```python
from build123d import *

# Parameters (mm, degrees)
SKETCH1_W                       = 45
SKETCH1_H                       = 20
SKETCH1_R                       = 4.9235
BOSS_EXTRUDE1_DEPTH             = 12.7
TAP_DRILL_FOR_M3X0_5_TAP1_D     = 2.584625
TAP_DRILL_FOR_M3X0_5_TAP1_DEPTH = 10
TAP_DRILL_FOR_M3X0_5_TAP1_TIP   = 0.776499689
FILLET1_R                       = 2
CHAMFER1_SIZE                   = 0.5


with BuildPart() as part:
    # Sketch1 → Boss-Extrude1 (new body)
    with BuildSketch(Plane.XY):
        with Locations((5.818965517, -6.284482759)):
            Rectangle(SKETCH1_W, SKETCH1_H)
        with Locations((-6.681034483, -8.784482759)):
            Circle(SKETCH1_R, mode=Mode.SUBTRACT)
        with Locations((18.318965517, -8.784482759)):
            Circle(SKETCH1_R, mode=Mode.SUBTRACT)
    extrude(amount=BOSS_EXTRUDE1_DEPTH)

    # Tap Drill for M3x0.5 Tap1
    with Locations(Plane.XY.offset(12.7)):
        with Locations((5.818965517, -6.284482759), (5.818965517, -11.284482759)):
            Hole(TAP_DRILL_FOR_M3X0_5_TAP1_D / 2, depth=TAP_DRILL_FOR_M3X0_5_TAP1_DEPTH)
            with Locations((0, 0, -(TAP_DRILL_FOR_M3X0_5_TAP1_DEPTH + TAP_DRILL_FOR_M3X0_5_TAP1_TIP / 2))):  # 118° drill point
                Cone(0, TAP_DRILL_FOR_M3X0_5_TAP1_D / 2, TAP_DRILL_FOR_M3X0_5_TAP1_TIP, mode=Mode.SUBTRACT)

    # Fillet1
    fillet1_edges = [part.edges().sort_by_distance(p)[0] for p in [
        (-16.681034483, 3.715517241, 6.35),
        (28.318965517, 3.715517241, 6.35),
        (28.318965517, -16.284482759, 6.35),
        (-16.681034483, -16.284482759, 6.35),
    ]]
    fillet(fillet1_edges, radius=FILLET1_R)

    # Sketch8 → Tap Drill for M3x0.5 Tap2 (revolve, cut)
    with BuildSketch(Plane(origin=(-16.681034483, -3.784482759, 2.5), x_dir=(0, 0, 1), z_dir=(0, 1, 0))):
        Polygon((0, 0), (0, 5.776499689), (1.2923125, 5), (1.2923125, 0), align=None)
    tap_drill_for_m3x0_5_tap2 = revolve(axis=Axis((-23.031034483, -3.784482759, 2.5), (1, 0, 0)), mode=Mode.SUBTRACT)

    # Mirror3: Tap Drill for M3x0.5 Tap2 across plane
    add(tap_drill_for_m3x0_5_tap2.mirror(Plane(origin=(5.818965517, 0, 0), x_dir=(0, 0, 1), z_dir=(1, 0, 0))), mode=Mode.SUBTRACT)

    # Chamfer1
    chamfer1_edges = [part.edges().sort_by_distance(p)[0] for p in [
        (-16.681034483, -3.784482759, 1.2076875),
        (28.318965517, -3.784482759, 1.2076875),
    ]]
    chamfer(chamfer1_edges, length=CHAMFER1_SIZE)


solid = part.part
```
CAD build for the part. Positions are in the model's coordinates, mm. A direction names the side the tool comes from. Coordinates: 2 decimals unless noted, no trailing zeros. Write each loop counter-clockwise with the first axis right and the second up, starting at its lowest first coordinate (ties: lowest second). Pieces come first, ordered by that corner, then holes.
(1) Two-plate mould, pull along Y, no slides. Class faces 5 (the face through (5.77, -11.504, 2.058)), 6 (the face through (-16.111, 3.114, 6.439)), 7 (the face through (6, -4, 12.7)): +Y half, -Y half, draft (parallel to the pull), parting line (faces both ways), or undercut.
(2) Cut at A-A, the plane z = 9.75. List the corners of the cut face in (x, y).
(3) Flat gauge pins, fed straight in: pin 1 (2.5 mm diameter, centred on y = -3.78, z = 2.5, fed in from +X); pin 2 (3.5 mm diameter, centred on y = -3.78, z = 2.5, fed in from -X). Where does each tip first touch, or does it go through?
(4) Cut at C-C, the plane x = -13. List the corners of the cut face in (y, z).
(5) Cut at D-D, the plane y = -7. Count the separate pieces of the cut face and the enclosed holes in it, and give its area (3 significant figures).
(6) Cut at B-B, the plane x = -5. List the corners of the cut face in (y, z), and give its area (3 significant figures).
(7) Drill centre lines: probe 1 along X at (y, z) = (-13.25, 11.75); probe 2 along X at (y, z) = (-9.5, 12.25); probe 3 along Y at (x, z) = (5.5, 11.25). Where is each one in solid material? Low to high.
(8) 3-axis set-ups, long thin cutter, end or side, ignore diameter. For faces 1 (the face through (7.11, -11.23, 7.63)), 2 (the face through (27.718, 3.145, 6.439)), 3 (the face through (25.6, -2.523, 2.22)), 4 (the face through (-13.963, -2.523, 2.22)): which of +Z, -Z, +X, -X, +Y, -Y reach the whole face in a straight line?
Geometry says:
1. face 5: undercut
1. face 6: +Y half
1. face 7: draft
2. outline: (-16.68, -14.28) arc R2 ccw to (-14.68, -16.28) - (26.32, -16.28) arc R2 ccw to (28.32, -14.28) - (28.32, 1.72) arc R2 ccw to (26.32, 3.72) - (-14.68, 3.72) arc R2 ccw to (-16.68, 1.72) - close; hole circle Ø9.85 at (-6.68, -8.78); hole circle Ø2.58 at (5.82, -11.28); hole circle Ø2.58 at (5.82, -6.28); hole circle Ø9.85 at (18.32, -8.78)
3. pin 1: stops at x = 23.3
3. pin 2: stops at x = -16.64
4. outline: (-16.28, 0) - (3.72, 0) - (3.72, 12.7) - (-16.28, 12.7) - close; hole circle Ø2.58 at (-3.78, 2.5)
5. separate pieces: 3
5. enclosed holes: 0
5. area: 316 mm2
6. outline: (-16.28, 0) - (-13.41, 0) - (-13.41, 12.7) - (-16.28, 12.7) - close; (-4.16, 0) - (3.72, 0) - (3.72, 12.7) - (-4.16, 12.7) - close
6. area: 136 mm2
7. probe 1: x = -16.68 to -8.75, -4.61 to 16.25, 20.39 to 28.32
7. probe 2: x = -16.68 to -11.55, -1.81 to 13.45, 23.19 to 28.32
7. probe 3: y = -16.28 to -12.54, -10.03 to -7.54, -5.03 to 3.72
8. face 1: +Z
8. face 2: +Z, -Z, +X, +Y
8. face 3: +X
8. face 4: -X
